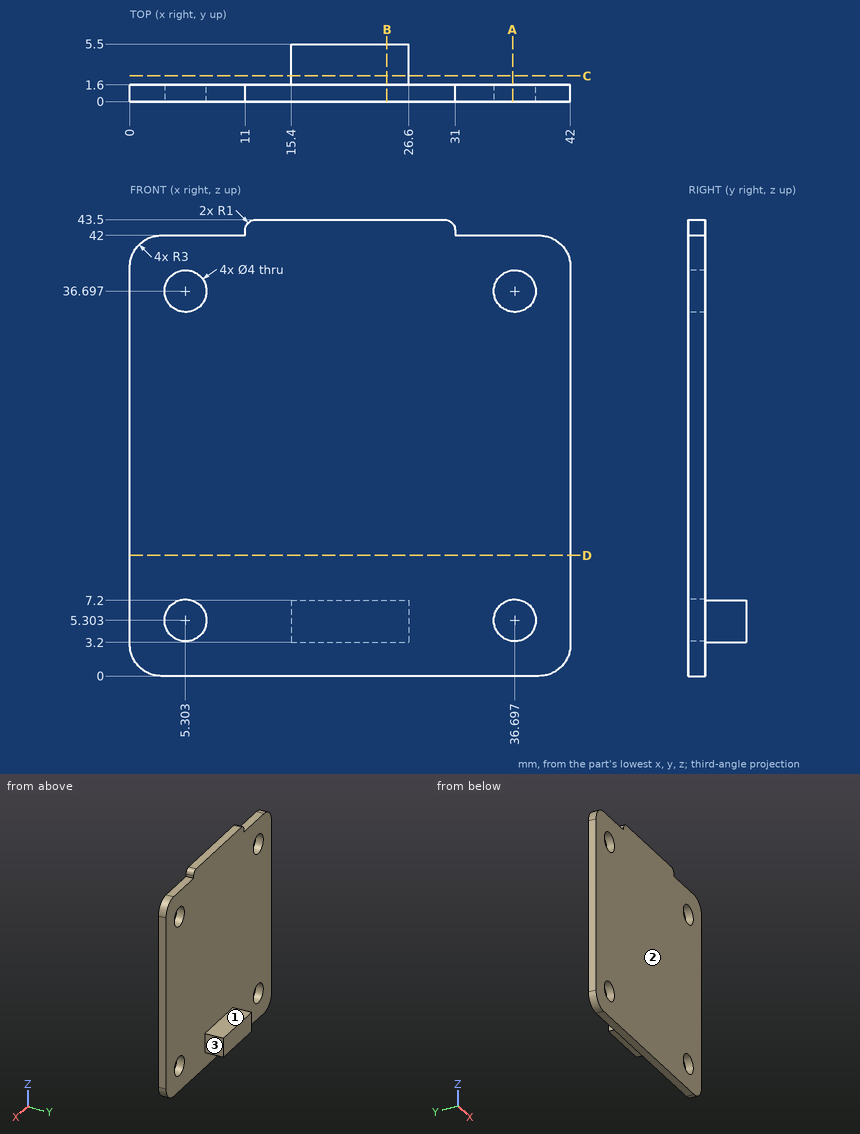
Job drawing, mm, ordinate dimensions from the low corner. One solid piece. A direction names the side the tool comes from. Round coordinates to 2 decimals unless told otherwise and drop trailing zeros. Loops run counter-clockwise (first coordinate to the right, second up) from the corner with the lowest first, then second, coordinate; pieces in that order, holes last.
(1) Cut at D-D (z = 11.5). Give the cut face in (x, y).
(2) Drop flat-ended pins along their axis: pin 1 (5 mm diameter, centred on x = 5.3, z = 36.7, fed in from +Y); pin 2 (1.2 mm diameter, centred on y = 3, z = 6, fed in from -X); pin 3 (0.5 mm diameter, centred on x = 35.5, y = 0.5, fed in from +Z). Give the stop position or say it passes through.
(3) Wall check: line 1 along Z through (x, y) = (38, 1.55) (1 decimal); line 2 along X through (y, z) = (4, 3.5); line 3 along Z through (x, y) = (19.5, 2.25). Give the ranges that are in metal, low to high.
(4) Cut at C-C (y = 2.45). Give the cut face in (x, z), plus the area to 3 significant figures.
(5) Which spindle directions (+Z, -Z, +X, -X, +Y, -Y) get a long thin tool onto all of the face, cutting with end or side? Do the marked faces 1, 2 and 3. Say none if no direction does.
(6) Cut at A-A (x = 36.5). Give the cut face in (y, z).
(7) Cut at B-B (x = 24.5). Give the cut face in (y, z).
Findings below:
1. outline: (0, 0) - (42, 0) - (42, 1.6) - (0, 1.6) - close
2. pin 1: stops at y = 1.6
2. pin 2: stops at x = 15.4
2. pin 3: stops at z = 42
3. line 1: z = 0 to 3.8, 6.8 to 35.2, 38.2 to 42
3. line 2: x = 15.4 to 26.6
3. line 3: z = 3.2 to 7.2
4. outline: (15.4, 3.2) - (26.6, 3.2) - (26.6, 7.2) - (15.4, 7.2) - close
4. area: 44.8 mm2
5. face 1: +Z, +X, -X, +Y
5. face 2: +Z, -Z, +X, -X, -Y
5. face 3: +Z, -Z, +X, +Y
6. outline: (0, 0) - (1.6, 0) - (1.6, 3.31) - (0, 3.31) - close; (0, 7.29) - (1.6, 7.29) - (1.6, 34.71) - (0, 34.71) - close; (0, 38.69) - (1.6, 38.69) - (1.6, 42) - (0, 42) - close
7. outline: (0, 0) - (1.6, 0) - (1.6, 3.2) - (5.5, 3.2) - (5.5, 7.2) - (1.6, 7.2) - (1.6, 43.5) - (0, 43.5) - close
